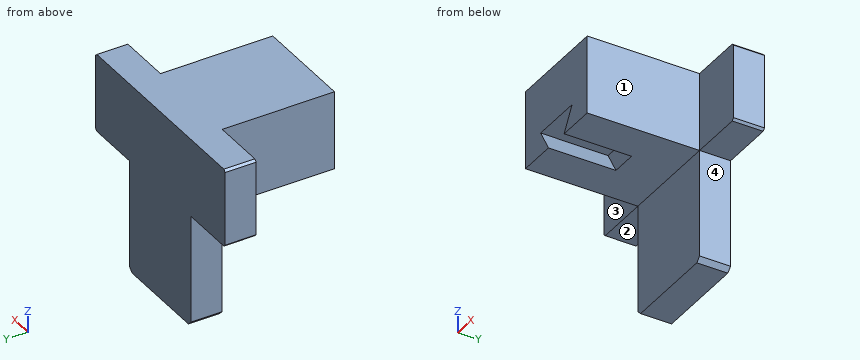
from build123d import *

# Parameters (mm, degrees)
F0_W     = 94.91
F0_H     = 35
F1_DEPTH = 13.78
F2_SIZE  = 1
F3_W     = 45.17
F3_H     = 35
F4_DEPTH = 50
F5_W     = 45.17
F5_H     = 13.78
F6_DEPTH = 50
F8_DEPTH = 30
F9_SIZE  = 2


with BuildPart() as f1:
    # F0 (on Front) → F1 (new body)
    with BuildSketch(Plane.XZ):
        with Locations((-0.477387, -10.428106)):
            Rectangle(F0_W, F0_H)
    extrude(amount=F1_DEPTH)

    # F2
    f2_edges = [f1.edges().sort_by_distance(p)[0] for p in [
        (-47.932387, -6.89, -27.928106),
        (46.977613, -6.89, -27.928106),
        (46.977613, -6.89, 7.071894),
        (-47.932387, -6.89, 7.071894),
    ]]
    chamfer(f2_edges, length=F2_SIZE)

    # F3 (on face) → F4 (join)
    with BuildSketch(Plane.XZ.offset(13.78)):
        with Locations((-0.477387, -10.428106)):
            Rectangle(F3_W, F3_H)
    extrude(amount=F4_DEPTH)

    # F5 (on face) → F6 (join)
    with BuildSketch(Plane(origin=(0, 0, -27.928106), x_dir=(1, 0, 0), z_dir=(0, 0, -1))):
        with Locations((-0.477387, 6.89)):
            Rectangle(F5_W, F5_H)
    extrude(amount=F6_DEPTH)

    # F7 (on face) → F8 (cut)
    with BuildSketch(Plane.XZ.offset(63.78)):
        Polygon((11.022613, -17.928106), (-11.977387, -17.928106), (-6.203884, -27.928106), (5.249111, -27.928106), align=None)
    extrude(amount=-F8_DEPTH, mode=Mode.SUBTRACT)

    # F9
    f9_edges = [f1.edges().sort_by_distance(p)[0] for p in [
        (-23.062387, -6.89, -77.928106),
        (22.107613, -6.89, -77.928106),
    ]]
    chamfer(f9_edges, length=F9_SIZE)


solid = f1.part
Work out the finished part from the listing and answer in its coordinate system (mm). Face numbers are marked on the shaded views. A direction names the side the tool comes from. Round coordinates to 2 decimals unless told otherwise and drop trailing zeros. Write each loop counter-clockwise with the first axis right and the second up, starting at its lowest first coordinate (ties: lowest second). Pieces come first, ordered by that corner, then holes.
1) A cutting plane is placed at A-A (x = 14). Give the vertices of the cut face in (y, z).
2) Straight lines are drawn through the part: line 1 (Z direction, x = -8, y = -22); line 2 (Z direction, x = -5, y = -58.5); line 3 (X direction, y = -50, z = -15). For each, find the intervals that lie inside material, in ascending order.
3) A cutting plane is placed at C-C (z = -6). Give the vertices of the cut face in (x, y).
4) Given pin 1 Ø11.5 at (x, y) = (-3, -51.5) entering from -Z; pin 2 Ø7 at (y, z) = (-4, -42.5) entering from -X; pin 3 Ø2 at (x, z) = (-1, -31.5) entering from -Y, each flat-ended and moving along its own axis, determine where each tip first touches the part or whether it passes through.
5) A cutting plane is placed at B-B (y = -46.5). Give the vertices of the cut face in (x, z).
6) A cutting plane is placed at D-D (y = -31). Give the vertices of the cut face in (x, z).
7) A tool of negligible diameter and unlimited length cuts with its end or side. For the marked faces 1, 2, 3 and 4, from which of +Z, -Z, +X, -X, +Y, -Y can it reach the whole face along a straight path? Write none if from no direction.
Completed:
1. outline: (-63.78, -27.93) - (-13.78, -27.93) - (-13.78, -77.93) - (0, -77.93) - (0, 7.07) - (-63.78, 7.07) - close
2. line 1: z = -27.93 to 7.07
2. line 2: z = -17.93 to 7.07
2. line 3: x = -23.06 to 22.11
3. outline: (-47.93, -13.78) - (-23.06, -13.78) - (-23.06, -63.78) - (22.11, -63.78) - (22.11, -13.78) - (46.98, -13.78) - (46.98, 0) - (-47.93, 0) - close
4. pin 1: stops at z = -27.93
4. pin 2: stops at x = -23.06
4. pin 3: stops at y = -13.78
5. outline: (-23.06, -27.93) - (-6.2, -27.93) - (-11.98, -17.93) - (11.02, -17.93) - (5.25, -27.93) - (22.11, -27.93) - (22.11, 7.07) - (-23.06, 7.07) - close
6. outline: (-23.06, -27.93) - (22.11, -27.93) - (22.11, 7.07) - (-23.06, 7.07) - close
7. face 1: +Z, -Z, +X, -Y
7. face 2: -Z, -X, +Y, -Y
7. face 3: +Z, -Z, -X, -Y
7. face 4: -Z, +X, +Y, -Y
